from build123d import *

# Parameters (mm, degrees)
SKETCH1_W             = 200
SKETCH1_H             = 100
BOSS_EXTRUDE1_DEPTH   = 6.35
CHAMFER1_SIZE         = 5
CHAMFER1_SIZE2        = 20
FILLET1_R             = 10
F_3_0MM_DOWEL_HOLE1_D = 3
M8_CLEARANCE_HOLE1_D  = 9
F_6_0MM_DOWEL_HOLE1_D = 7


with BuildPart() as part:
    # Sketch1 → Boss-Extrude1 (new body)
    with BuildSketch(Plane(origin=(0, 0, 0), x_dir=(1, 0, 0), z_dir=(0, 1, 0))):
        Rectangle(SKETCH1_W, SKETCH1_H)
    extrude(amount=BOSS_EXTRUDE1_DEPTH)

    # Chamfer1
    chamfer1_edges = [part.edges().sort_by_distance(p)[0] for p in [
        (-100, 6.35, 0),
    ]]
    chamfer1_side = [part.faces().sort_by_distance(p)[0] for p in [
        (-100, 3.175, 0),
    ]]
    chamfer(chamfer1_edges, length=CHAMFER1_SIZE, length2=CHAMFER1_SIZE2, reference=chamfer1_side[0])

    # Fillet1
    fillet1_edges = [part.edges().sort_by_distance(p)[0] for p in [
        (-80, 6.35, 0),
        (-100, 0.675, 50),
        (-100, 0.675, -50),
        (100, 3.175, 50),
        (100, 3.175, -50),
    ]]
    fillet(fillet1_edges, radius=FILLET1_R)

    # Ø3.0mm Dowel Hole1 (through all)
    with Locations(Plane(origin=(0, 6.35, 0), x_dir=(1, 0, 0), z_dir=(0, 1, 0))):
        with Locations((-57, 0), (57, 0)):
            Hole(F_3_0MM_DOWEL_HOLE1_D / 2)

    # M8 Clearance Hole1 (through all)
    with Locations(Plane(origin=(0, 6.35, 0), x_dir=(1, 0, 0), z_dir=(0, 1, 0))):
        with Locations((-60, 35), (80, -35), (-60, -35), (80, 35)):
            Hole(M8_CLEARANCE_HOLE1_D / 2)

    # Ø6.0mm Dowel Hole1 (through all)
    with Locations(Plane(origin=(0, 6.35, 0), x_dir=(1, 0, 0), z_dir=(0, 1, 0))):
        with Locations((-40.768943744, 25), (-40.768943744, -25)):
            Hole(F_6_0MM_DOWEL_HOLE1_D / 2)


solid = part.part
Build history of the part. All positions in model axes, mm. Round coordinates to 2 decimals unless told otherwise and drop trailing zeros. Loops run counter-clockwise (first coordinate to the right, second up) from the corner with the lowest first, then second, coordinate; pieces in that order, holes last. Notation, with made-up numbers: (-15, -38.5) -> (37, -38.5) arc R23 cw to (37, -26.5) -> close; hole circle Ø5 at (62.25, 85). An arc over 180 degrees is marked (long way). Answer in a Markdown table with one row per item.
Item 1: Saw through at C-C (y = 2.5). State how many separate pieces and enclosed holes the cut face has, and give its area (3 significant figures).
Answers below:
| item | result |
|---|---|
| separate pieces | 1 |
| enclosed holes | 8 |
| area | 19,100 mm² |
Item 2: Mould opens along Z. For faces 1 (the cylindrical face through (80.98, 3.13, -30.61)), 2 (the flat face through (-1, 3, -50)), 3 (the cylindrical face through (-44.107, 3.131, 23.949)), 4 (the flat face through (9, 6.35, -1)) say: +Z half, -Z half, draft (parallel to the pull), parting line (faces both ways), or undercut.
Answers below:
| item | result |
|---|---|
| face 1 | undercut |
| face 2 | -Z half |
| face 3 | undercut |
| face 4 | draft |
Item 3: Saw through at A-A (x = 80). Write the cut outline in (y, z), and give its area (3 significant figures).
Answers below:
| item | result |
|---|---|
| outline | (0, -50) -> (6.35, -50) -> (6.35, -39.5) -> (0, -39.5) -> close; (0, -30.5) -> (6.35, -30.5) -> (6.35, 30.5) -> (0, 30.5) -> close; (0, 39.5) -> (6.35, 39.5) -> (6.35, 50) -> (0, 50) -> close |
| area | 521 mm² |
Item 4: Saw through at B-B (z = 35). Write the cut outline in (x, y), and give its area (3 significant figures).
Answers below:
| item | result |
|---|---|
| outline | (-100, 0) -> (-64.5, 0) -> (-64.5, 6.35) -> (-78.77, 6.35) arc R10 ccw to (-81.19, 6.05) -> (-100, 1.35) -> close; (-55.5, 0) -> (75.5, 0) -> (75.5, 6.35) -> (-55.5, 6.35) -> close; (84.5, 0) -> (100, 0) -> (100, 6.35) -> (84.5, 6.35) -> close |
| area | 1,110 mm² |
Item 5: Pin check, flat tip, straight feed: pin 1 (8 mm diameter, centred on x = 80, z = -35, fed in from -Y). Stop position of the tip, or through.
Answers below:
| item | result |
|---|---|
| pin 1 | passes through |
Item 6: Drill centre lines: L1, parallel to Z at x = -60, y = 2.5; L2, parallel to Z at x = 57, y = 4.5; L3, parallel to Y at x = -86, z = 23. Where is each one in solid material? Low to high. Write a range as [from, to].
Answers below:
| item | result |
|---|---|
| L1 | z = [-50, -39.5], [-30.5, 30.5], [39.5, 50] |
| L2 | z = [-50, -1.5], [1.5, 50] |
| L3 | y = [0, 4.85] |
Item 7: Saw through at D-D (x = -62). Write the cut outline in (y, z).
Answers below:
| item | result |
|---|---|
| outline | (0, -50) -> (6.35, -50) -> (6.35, -39.03) -> (0, -39.03) -> close; (0, -30.97) -> (6.35, -30.97) -> (6.35, 30.97) -> (0, 30.97) -> close; (0, 39.03) -> (6.35, 39.03) -> (6.35, 50) -> (0, 50) -> close |
